```python
from build123d import *

# Parameters (mm, degrees)
SKETCH1_R           = 39.75
BOSS_EXTRUDE1_DEPTH = 10
CUT_EXTRUDE4_DEPTH  = 10
CHAMFER1_SIZE       = 2
CHAMFER2_SIZE       = 2
CHAMFER3_SIZE       = 2
CHAMFER4_SIZE       = 2


with BuildPart() as part:
    # Sketch1 → Boss-Extrude1 (new body)
    with BuildSketch(Plane(origin=(0, 0, 0), x_dir=(1, 0, 0), z_dir=(0, 1, 0))):
        with Locations(Location((0, 0, 0), (0, 0, 270))):
            Circle(SKETCH1_R)
    extrude(amount=BOSS_EXTRUDE1_DEPTH)

    # Sketch2 → Cut-Extrude4 (cut)
    with BuildSketch(Plane(origin=(0, 10, 0), x_dir=(1, 0, 0), z_dir=(0, 1, 0))):
        with BuildLine():
            Line((30.35, 0), (37.75, 0))
            ThreePointArc((37.75, 0), (34.876452352, 14.446299572), (26.69328099, 26.69328099))
            Line((26.69328099, 26.69328099), (21.460690809, 21.460690809))
            ThreePointArc((21.460690809, 21.460690809), (0, 30.35), (-21.460690809, 21.460690809))
            Line((-21.460690809, 21.460690809), (-24.076985899, 24.076985899))
            ThreePointArc((-24.076985899, 24.076985899), (-31.458098082, 13.030370872), (-34.05, 0))
            Line((-34.05, 0), (-30.35, 0))
            ThreePointArc((-30.35, 0), (0, -30.35), (30.35, 0))
        make_face()
    extrude(amount=-CUT_EXTRUDE4_DEPTH, mode=Mode.SUBTRACT)

    # Chamfer1
    chamfer1_edges = [part.edges().sort_by_distance(p)[0] for p in [
        (34.05, 0, 0),
    ]]
    chamfer(chamfer1_edges, length=CHAMFER1_SIZE)

    # Chamfer2
    chamfer2_edges = [part.edges().sort_by_distance(p)[0] for p in [
        (-32.2, 0, 0),
    ]]
    chamfer(chamfer2_edges, length=CHAMFER2_SIZE)

    # Chamfer3
    chamfer3_edges = [part.edges().sort_by_distance(p)[0] for p in [
        (24.076985899, 10, -24.076985899),
    ]]
    chamfer(chamfer3_edges, length=CHAMFER3_SIZE)

    # Chamfer4
    chamfer4_edges = [part.edges().sort_by_distance(p)[0] for p in [
        (-22.768838354, 10, -22.768838354),
    ]]
    chamfer(chamfer4_edges, length=CHAMFER4_SIZE)


solid = part.part
```
Verification items for the finished model (mm, model axes). A direction names the side the tool comes from. Give positions to 0.01 mm unless a question says otherwise; leave off trailing zeros. Order: outer loops, then holes, each group sorted by start corner. A loop starts at its lowest first (then second) coordinate and runs counter-clockwise, first axis right, second up. Notation, with made-up numbers: M 55.25,45 L 87.25,45 A19 cw 87.25,64 Z; hole C 42,64 d3. An arc over 180 degrees is marked long. Return JSON: item names as keys, results as strings. Group by question number.
1) Scan lines: line 1 (X direction, y = 7.5, z = 0.5); line 2 (X direction, y = 8, z = -18); line 3 (Z direction, x = 23, y = 1.75). Record each from-to range of solid material in increasing order.
2) Section check D-D on x = 31.5. Record the cut outline in (y, z).
3) Go/stop test with flat-tipped pins: pin 1 Ø5 at (y, z) = (8.5, 22) entering from +X; pin 2 Ø1 at (y, z) = (7, -7) entering from -X; pin 3 Ø3 at (x, y) = (-19.5, 4.5) entering from +Z. Record where each tip stops, or that it passes through.
4) Section check B-B on z = 25. Record the cut outline in (x, y), and give its area (3 significant figures).
5) Mould release check, pull along X, two halves, no side actions. Record for faces 4 (the face through (-20.4, 10, 23.4)), 5 (the face through (34, 6, 0)), 6 (the face through (39.412, 4.93, -5.175)): pulls with the +X half, pulls with the -X half, needs draft (parallel to the pull), parting line crosses it, or undercut.
6) Section check C-C on y = 5. Record the cut outline in (x, z).
7) Access from +Z, -Z, +X, -X, +Y, -Y to the whole of each face (thin tool, end or side, straight path). Record for faces 1 (the face through (34, 1, 1)), 2 (the face through (-0.667, 5.07, 30.343)), 3 (the face through (23.39, 8.99, -24.79)).
8) Section check A-A on x = 0. Record the cut outline in (y, z).
Answer block:
{
 "1": {"line 1": "x = -39.75 to -30.35, 30.35 to 39.75", "line 2": "x = -35.44 to -28.9, 33.18 to 35.44", "line 3": "z = -32.42 to -23, 19.8 to 32.42"},
 "2": {"outline": "M 0,-24.24 L 10,-24.24 L 10,-20.8 L 0,-20.8 Z; M 0,2 L 2,0 L 10,0 L 10,24.24 L 0,24.24 Z"},
 "3": {"pin 1": "stops at x = 34.64", "pin 2": "stops at x = -39.21", "pin 3": "stops at z = 35.44"},
 "4": {"outline": "M -30.9,0 L -17.21,0 L -17.21,10 L -30.9,10 Z; M 17.21,0 L 30.9,0 L 30.9,10 L 17.21,10 Z", "area": "274 mm^2"},
 "5": {"face 4": "needs draft", "face 5": "undercut", "face 6": "parting line crosses it"},
 "6": {"outline": "C 0,0 d79.5; hole M -34.05,0 A34.05 ccw -24.08,-24.08 L -21.46,-21.46 A30.35 ccw 21.46,-21.46 L 26.69,-26.69 A37.75 ccw 37.75,0 L 30.35,0 A30.35 ccw -30.35,0 Z"},
 "7": {"face 1": "-Y", "face 2": "+Y, -Y", "face 3": "+Y"},
 "8": {"outline": "M 0,-39.75 L 10,-39.75 L 10,-30.35 L 0,-30.35 Z; M 0,30.35 L 10,30.35 L 10,39.75 L 0,39.75 Z"}
}
